from build123d import *

# Parameters (mm, degrees)
SKETCH_1_W        = 2.54
SKETCH_1_H        = 2.54
EXTRUDE_1_DEPTH   = 2.54
SKETCH_2_W        = 0.67
SKETCH_2_H        = 0.67
EXTRUDE_1_2_DEPTH = 2.54
SKETCH_3_W        = 0.67
SKETCH_3_H        = 0.67
EXTRUDE_2_DEPTH   = 19.92
FILLET_1_R        = 0.2


with BuildPart() as part:
    # 草图1 → Extrude 1 (new body)
    with BuildSketch(Plane.XY):
        Rectangle(SKETCH_1_W, SKETCH_1_H)
    extrude(amount=EXTRUDE_1_DEPTH)

    # 草图2 → Extrude 1 2 (add)
    with BuildSketch(Plane(origin=(0, 0, 0), x_dir=(-1, 0, 0), z_dir=(0, 0, -1))):
        Rectangle(SKETCH_2_W, SKETCH_2_H)
    extrude(amount=EXTRUDE_1_2_DEPTH)

    # 草图3 → 凸台-拉伸2 (add)
    with BuildSketch(Plane.XY.offset(2.54)):
        Rectangle(SKETCH_3_W, SKETCH_3_H)
    extrude(amount=EXTRUDE_2_DEPTH)

    # 圆角1
    fillet_1_edges = [part.edges().sort_by_distance(p)[0] for p in [
        (-1.27, 1.27, 1.27),
        (1.27, 1.27, 1.27),
        (1.27, -1.27, 1.27),
        (-1.27, -1.27, 1.27),
    ]]
    fillet(fillet_1_edges, radius=FILLET_1_R)


solid = part.part
Check sheet for the modelled part. Datum: model origin and axes. Units: mm. Give positions to 0.01 mm unless a question says otherwise; leave off trailing zeros. Write each loop counter-clockwise with the first axis right and the second up, starting at its lowest first coordinate (ties: lowest second). Pieces come first, ordered by that corner, then holes. Notation, with made-up numbers: (21, 71) -> (38, 71) arc R21 cw to (38, 96) -> close; hole circle Ø3 at (33, -39.75). An arc over 180 degrees is marked (long way). Write item = value, one per line.
Item 1: Sectioned sample at A-A on x = 0. Record the boundary of the cut face in (y, z) (3 decimals).
Output:
outline = (-1.27, 0) -> (-0.335, 0) -> (-0.335, -2.54) -> (0.335, -2.54) -> (0.335, 0) -> (1.27, 0) -> (1.27, 2.54) -> (0.335, 2.54) -> (0.335, 22.46) -> (-0.335, 22.46) -> (-0.335, 2.54) -> (-1.27, 2.54) -> close
Item 2: Scan lines: probe 1 along Z at (x, y) = (-0.5, 0.8); probe 2 along X at (y, z) = (-0.3, 9.75) (3 decimals). Record each from-to range of solid material in increasing order. Write a range as from..to.
Output:
probe_1 = 0..2.54
probe_2 = -0.335..0.335
Item 3: Sectioned sample at B-B on z = 16.5. Record the boundary of the cut face in (x, y) (3 decimals).
Output:
outline = (-0.335, -0.335) -> (0.335, -0.335) -> (0.335, 0.335) -> (-0.335, 0.335) -> close
Item 4: Gauge pin test, flat ends, axial feed: pin 1 (0.7 mm diameter, centred on y = 0, z = 11.5, fed in from +X) (3 decimals); pin 2 (0.5 mm diameter, centred on x = 0, z = 11.5, fed in from +Y) (3 decimals); pin 3 (0.7 mm diameter, centred on y = 0, z = -1, fed in from -X) (3 decimals). Record the tip position at first contact, or that the pin passes through.
Output:
pin_1 = 0.335
pin_2 = 0.335
pin_3 = -0.335
Item 5: Sectioned sample at C-C on y = -0.6. Record the boundary of the cut face in (x, z), and give its area (3 significant figures).
Output:
outline = (-1.27, 0) -> (1.27, 0) -> (1.27, 2.54) -> (-1.27, 2.54) -> close
area = 6.45 mm^2
